```python
from build123d import *

# Parameters (mm, degrees)
F0_W      = 914.4
F0_H      = 914.4
F1_DEPTH  = 177.8
F2_W      = 609.6
F2_H      = 609.6
F3_DEPTH  = 152.4
F6_DEPTH  = 50.8
F8_DEPTH  = 50.8
F9_W      = 914.4
F9_H      = 914.4
F9_W_2    = 863.6
F9_H_2    = 863.6
F10_DEPTH = 25.4


with BuildPart() as f1:
    # F0 (on Top) → F1 (new body)
    with BuildSketch(Plane.XY):
        with Locations((-0.90002447, 0.1499950886)):
            Rectangle(F0_W, F0_H)
    extrude(amount=F1_DEPTH)

    # F2 (on face) → F3 (cut)
    with BuildSketch(Plane(origin=(0, 0, 0), x_dir=(1, 0, 0), z_dir=(0, 0, -1))):
        with Locations((-0.90002447, -0.1499950886)):
            Rectangle(F2_W, F2_H)
    extrude(amount=-F3_DEPTH, mode=Mode.SUBTRACT)

    # F5 (on face) → F6 (cut)
    with BuildSketch(Plane.XZ.offset(457.0500049114)):
        with BuildLine():
            Line((380.09997553, 76.2), (393.5703597116, 62.7296158184))
            ThreePointArc((393.5703597116, 62.7296158184), (397.6998806243, 68.9098806134), (399.14997553, 76.2))
            ThreePointArc((399.14997553, 76.2), (397.6998806243, 83.4901193866), (393.5703597116, 89.6703841816))
            Line((393.5703597116, 89.6703841816), (380.09997553, 76.2))
        make_face()
        with BuildLine():
            Line((380.09997553, 76.2), (393.5703597116, 89.6703841816))
            ThreePointArc((393.5703597116, 89.6703841816), (380.09997553, 95.25), (366.6295913484, 89.6703841816))
            Line((366.6295913484, 89.6703841816), (380.09997553, 76.2))
        make_face()
        with BuildLine():
            ThreePointArc((366.6295913484, 89.6703841816), (361.04997553, 76.2), (366.6295913484, 62.7296158184))
            Line((366.6295913484, 62.7296158184), (380.09997553, 76.2))
            Line((380.09997553, 76.2), (366.6295913484, 89.6703841816))
        make_face()
        with BuildLine():
            ThreePointArc((366.6295913484, 62.7296158184), (380.09997553, 57.15), (393.5703597116, 62.7296158184))
            Line((393.5703597116, 62.7296158184), (380.09997553, 76.2))
            Line((380.09997553, 76.2), (366.6295913484, 62.7296158184))
        make_face()
        with BuildLine():
            Line((-381.90002447, 76.2), (-368.4296402884, 62.7296158184))
            ThreePointArc((-368.4296402884, 62.7296158184), (-364.3001193757, 68.9098806134), (-362.85002447, 76.2))
            ThreePointArc((-362.85002447, 76.2), (-364.3001193757, 83.4901193866), (-368.4296402884, 89.6703841816))
            Line((-368.4296402884, 89.6703841816), (-381.90002447, 76.2))
        make_face()
        with BuildLine():
            Line((-381.90002447, 76.2), (-368.4296402884, 89.6703841816))
            ThreePointArc((-368.4296402884, 89.6703841816), (-381.90002447, 95.25), (-395.3704086516, 89.6703841816))
            Line((-395.3704086516, 89.6703841816), (-381.90002447, 76.2))
        make_face()
        with BuildLine():
            ThreePointArc((-395.3704086516, 89.6703841816), (-400.95002447, 76.2), (-395.3704086516, 62.7296158184))
            Line((-395.3704086516, 62.7296158184), (-381.90002447, 76.2))
            Line((-381.90002447, 76.2), (-395.3704086516, 89.6703841816))
        make_face()
        with BuildLine():
            ThreePointArc((-395.3704086516, 62.7296158184), (-381.90002447, 57.15), (-368.4296402884, 62.7296158184))
            Line((-368.4296402884, 62.7296158184), (-381.90002447, 76.2))
            Line((-381.90002447, 76.2), (-395.3704086516, 62.7296158184))
        make_face()
    extrude(amount=-F6_DEPTH, mode=Mode.SUBTRACT)

    # F7 (on face) → F8 (cut)
    with BuildSketch(Plane.YZ.offset(456.29997553)):
        with BuildLine():
            Line((394.6203792702, 89.6703841816), (367.679610907, 62.7296158184))
            ThreePointArc((367.679610907, 62.7296158184), (388.4401144751, 58.6000949057), (400.1999950886, 76.2))
            ThreePointArc((400.1999950886, 76.2), (398.7499001829, 83.4901193866), (394.6203792702, 89.6703841816))
        make_face()
        with BuildLine():
            ThreePointArc((394.6203792702, 89.6703841816), (367.679610907, 89.6703841816), (367.679610907, 62.7296158184))
            Line((367.679610907, 62.7296158184), (394.6203792702, 89.6703841816))
        make_face()
        with BuildLine():
            Line((-394.320389093, 89.6703841816), (-367.3796207298, 62.7296158184))
            ThreePointArc((-367.3796207298, 62.7296158184), (-363.2500998171, 68.9098806134), (-361.8000049114, 76.2))
            ThreePointArc((-361.8000049114, 76.2), (-373.5598855249, 93.7999050943), (-394.320389093, 89.6703841816))
        make_face()
        with BuildLine():
            ThreePointArc((-394.320389093, 89.6703841816), (-394.320389093, 62.7296158184), (-367.3796207298, 62.7296158184))
            Line((-367.3796207298, 62.7296158184), (-394.320389093, 89.6703841816))
        make_face()
    extrude(amount=-F8_DEPTH, mode=Mode.SUBTRACT)

    # F9 (on face) → F10 (join)
    with BuildSketch(Plane.XY.offset(177.8)):
        with Locations((-0.90002447, 0.1499950886)):
            Rectangle(F9_W, F9_H)
        Rectangle(F9_W_2, F9_H_2, mode=Mode.SUBTRACT)
    extrude(amount=F10_DEPTH)


solid = f1.part
```
The listing builds one solid part. Answer for the finished solid, in the listing's coordinates (mm). A direction names the side the tool comes from. Give positions to 0.01 mm unless a question says otherwise; leave off trailing zeros. Order: outer loops, then holes, each group sorted by start corner. A loop starts at its lowest first (then second) coordinate and runs counter-clockwise, first axis right, second up. Notation, with made-up numbers: (48, 10) -> (76, 10) arc R34 cw to (76, 49) -> close; hole circle Ø3 at (6, 17). An arc over 180 degrees is marked (long way). One line per item, written item: value.
1) Determine the mould class of faces 1 (the flat face through (-5, 304.95, 75)), 2 (the flat face through (-7, -457.05, 100)), 3 (the flat face through (405.5, 381, 76)) for opening direction X: pulls with the +X half, pulls with the -X half, needs draft (parallel to the pull), parting line crosses it, or undercut.
Reported:
face 1: undercut
face 2: needs draft
face 3: pulls with the +X half
2) Find section C-C, the plane x = 61. Determine the outline of the cut face in (y, z), plus the area to 3 significant figures.
Reported:
outline: (-457.05, 0) -> (-304.65, 0) -> (-304.65, 152.4) -> (304.95, 152.4) -> (304.95, 0) -> (457.35, 0) -> (457.35, 203.2) -> (431.8, 203.2) -> (431.8, 177.8) -> (-431.8, 177.8) -> (-431.8, 203.2) -> (-457.05, 203.2) -> close
area: 71,000 mm^2
3) Find section A-A, the plane z = 141. Determine the outline of the cut face in (x, y), plus the area to 3 significant figures.
Reported:
outline: (-458.1, -457.05) -> (456.3, -457.05) -> (456.3, 457.35) -> (-458.1, 457.35) -> close; hole (-305.7, -304.65) -> (303.9, -304.65) -> (303.9, 304.95) -> (-305.7, 304.95) -> close
area: 465,000 mm^2
4) A tool of negligible diameter and unlimited length cuts with its end or side. For faces 4 (the flat face through (456.3, -6, 100)), 5 (the flat face through (-5, -304.65, 75)), 6 (the flat face through (431.8, -6, 190)), 7 (the flat face through (405.5, -381, 76)), 8 (the flat face through (-382, -406.25, 76)), from which of +Z, -Z, +X, -X, +Y, -Y can it reach the whole face along a straight path? Write none if from no direction.
Reported:
face 4: +Z, -Z, +X, +Y, -Y
face 5: -Z
face 6: +Z
face 7: +X
face 8: -Y
5) Find the intervals of material crossed by line 1 (Y direction, x = -240.5, z = 106.5); line 2 (Y direction, x = -106, z = 179); line 3 (X direction, y = -302.5, z = 135.5), in increasing order.
Reported:
line 1: y = -457.05 to -304.65, 304.95 to 457.35
line 2: y = -457.05 to -431.8, 431.8 to 457.35
line 3: x = -458.1 to -305.7, 303.9 to 456.3
6) Flat-ended cylindrical pins translate along their axes: P1, Ø5, axis at x = 248, y = 51, coming from the +Z side; P2, Ø11.5, axis at y = 379, z = 70, coming from the +X side; P3, Ø10, axis at x = -33, y = 247.5, coming from the -Z side. Find the tip coordinate at first contact, or state that the pin passes through.
Reported:
P1: stops at z = 177.8
P2: stops at x = 405.5
P3: stops at z = 152.4
7) Find section B-B, the plane y = 65.5. Determine the outline of the cut face in (x, z).
Reported:
outline: (-458.1, 0) -> (-305.7, 0) -> (-305.7, 152.4) -> (303.9, 152.4) -> (303.9, 0) -> (456.3, 0) -> (456.3, 203.2) -> (431.8, 203.2) -> (431.8, 177.8) -> (-431.8, 177.8) -> (-431.8, 203.2) -> (-458.1, 203.2) -> close
